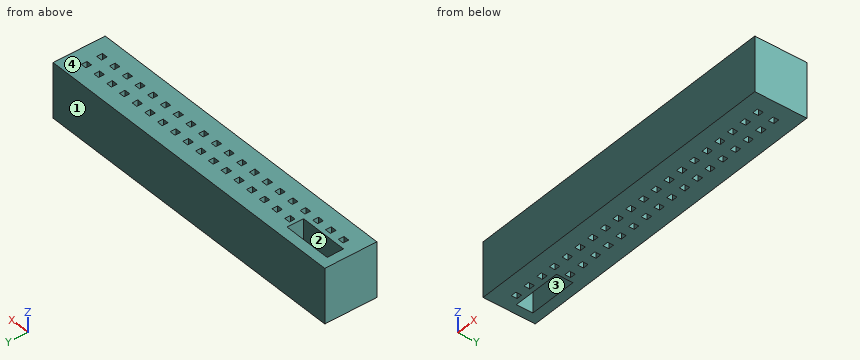
from build123d import *

# Parameters (mm, degrees)
F0_W     = 54.26
F0_H     = 8.54
F0_W_2   = 0.93338
F0_H_2   = 0.93338
F1_DEPTH = 9
F2_W     = 8
F2_H     = 2.7
F3_DEPTH = 25


with BuildPart() as f1:
    # F0 (on Top) → F1 (new body)
    with BuildSketch(Plane.XY):
        with Locations((24.13, 1.27)):
            Rectangle(F0_W, F0_H)
        Rectangle(F0_W_2, F0_H_2, mode=Mode.SUBTRACT)
        with Locations((2.54, 0)):
            Rectangle(F0_W_2, F0_H_2, mode=Mode.SUBTRACT)
        with Locations((5.08, 0)):
            Rectangle(F0_W_2, F0_H_2, mode=Mode.SUBTRACT)
        with Locations((7.62, 0)):
            Rectangle(F0_W_2, F0_H_2, mode=Mode.SUBTRACT)
        with Locations((10.16, 0)):
            Rectangle(F0_W_2, F0_H_2, mode=Mode.SUBTRACT)
        with Locations((12.7, 0)):
            Rectangle(F0_W_2, F0_H_2, mode=Mode.SUBTRACT)
        with Locations((15.24, 0)):
            Rectangle(F0_W_2, F0_H_2, mode=Mode.SUBTRACT)
        with Locations((17.78, 0)):
            Rectangle(F0_W_2, F0_H_2, mode=Mode.SUBTRACT)
        with Locations((20.32, 0)):
            Rectangle(F0_W_2, F0_H_2, mode=Mode.SUBTRACT)
        with Locations((22.86, 0)):
            Rectangle(F0_W_2, F0_H_2, mode=Mode.SUBTRACT)
        with Locations((25.4, 0)):
            Rectangle(F0_W_2, F0_H_2, mode=Mode.SUBTRACT)
        with Locations((27.94, 0)):
            Rectangle(F0_W_2, F0_H_2, mode=Mode.SUBTRACT)
        with Locations((30.48, 0)):
            Rectangle(F0_W_2, F0_H_2, mode=Mode.SUBTRACT)
        with Locations((33.02, 0)):
            Rectangle(F0_W_2, F0_H_2, mode=Mode.SUBTRACT)
        with Locations((35.56, 0)):
            Rectangle(F0_W_2, F0_H_2, mode=Mode.SUBTRACT)
        with Locations((38.1, 0)):
            Rectangle(F0_W_2, F0_H_2, mode=Mode.SUBTRACT)
        with Locations((40.64, 0)):
            Rectangle(F0_W_2, F0_H_2, mode=Mode.SUBTRACT)
        with Locations((43.18, 0)):
            Rectangle(F0_W_2, F0_H_2, mode=Mode.SUBTRACT)
        with Locations((45.72, 0)):
            Rectangle(F0_W_2, F0_H_2, mode=Mode.SUBTRACT)
        with Locations((48.26, 0)):
            Rectangle(F0_W_2, F0_H_2, mode=Mode.SUBTRACT)
        with Locations((0, 2.54)):
            Rectangle(F0_W_2, F0_H_2, mode=Mode.SUBTRACT)
        with Locations((2.54, 2.54)):
            Rectangle(F0_W_2, F0_H_2, mode=Mode.SUBTRACT)
        with Locations((5.08, 2.54)):
            Rectangle(F0_W_2, F0_H_2, mode=Mode.SUBTRACT)
        with Locations((7.62, 2.54)):
            Rectangle(F0_W_2, F0_H_2, mode=Mode.SUBTRACT)
        with Locations((10.16, 2.54)):
            Rectangle(F0_W_2, F0_H_2, mode=Mode.SUBTRACT)
        with Locations((12.7, 2.54)):
            Rectangle(F0_W_2, F0_H_2, mode=Mode.SUBTRACT)
        with Locations((15.24, 2.54)):
            Rectangle(F0_W_2, F0_H_2, mode=Mode.SUBTRACT)
        with Locations((17.78, 2.54)):
            Rectangle(F0_W_2, F0_H_2, mode=Mode.SUBTRACT)
        with Locations((20.32, 2.54)):
            Rectangle(F0_W_2, F0_H_2, mode=Mode.SUBTRACT)
        with Locations((22.86, 2.54)):
            Rectangle(F0_W_2, F0_H_2, mode=Mode.SUBTRACT)
        with Locations((25.4, 2.54)):
            Rectangle(F0_W_2, F0_H_2, mode=Mode.SUBTRACT)
        with Locations((27.94, 2.54)):
            Rectangle(F0_W_2, F0_H_2, mode=Mode.SUBTRACT)
        with Locations((30.48, 2.54)):
            Rectangle(F0_W_2, F0_H_2, mode=Mode.SUBTRACT)
        with Locations((33.02, 2.54)):
            Rectangle(F0_W_2, F0_H_2, mode=Mode.SUBTRACT)
        with Locations((35.56, 2.54)):
            Rectangle(F0_W_2, F0_H_2, mode=Mode.SUBTRACT)
        with Locations((38.1, 2.54)):
            Rectangle(F0_W_2, F0_H_2, mode=Mode.SUBTRACT)
        with Locations((40.64, 2.54)):
            Rectangle(F0_W_2, F0_H_2, mode=Mode.SUBTRACT)
        with Locations((43.18, 2.54)):
            Rectangle(F0_W_2, F0_H_2, mode=Mode.SUBTRACT)
        with Locations((45.72, 2.54)):
            Rectangle(F0_W_2, F0_H_2, mode=Mode.SUBTRACT)
        with Locations((48.26, 2.54)):
            Rectangle(F0_W_2, F0_H_2, mode=Mode.SUBTRACT)
    extrude(amount=F1_DEPTH)

    # F2 (on Top) → F3 (cut)
    with BuildSketch(Plane.XY):
        with Locations((2.54, 2.54)):
            Rectangle(F2_W, F2_H)
    extrude(amount=F3_DEPTH, mode=Mode.SUBTRACT)


solid = f1.part
Design review of the part built by this model. Coordinates are the model's own, in mm. Face numbers are marked on the shaded views. Give positions to 0.01 mm unless a question says otherwise; leave off trailing zeros. Use CSV: the item, a comma, the result in double quotes. Start each with the question number.
1. Wall thickness on L1, parallel to Y at x = 10, z = 2.5; L2, parallel to Y at x = 4, z = 8; L3, parallel to Y at x = 5, z = 3.75: over which ranges is each line inside the solid? List them lowest first.
2. Insertion check: P1, Ø1, axis at x = 42, y = -1, coming from the -Z side. The pin has a flat end and moves straight along its axis. Give the tip position at first contact, or say it passes through.
3. Add section A-A (y = 0). Count the separate pieces of the cut face and the enclosed holes in it, plus the area to 3 significant figures.
4. Draft analysis for pull direction Y (two halves, no side actions). For the marked faces 1, 2, 3 and 4, state which applies: released by +Y, released by -Y, zero draft, split by the parting line, or undercut.
Results found:
1,L1,"y = -3 to -0.47, 0.47 to 2.07, 3.01 to 5.54"
1,L2,"y = -3 to 1.19, 3.89 to 5.54"
1,L3,"y = -3 to -0.47, 0.47 to 1.19, 3.89 to 5.54"
2,P1,"stops at z = 0"
3,separate pieces,"21"
3,enclosed holes,"0"
3,area,"320 mm²"
4,face 1,"released by +Y"
4,face 2,"undercut"
4,face 3,"undercut"
4,face 4,"zero draft"
